Part model, mm, in its own coordinate system. A direction names the side the tool comes from. Give positions to 0.01 mm unless a question says otherwise; leave off trailing zeros. Order: outer loops, then holes, each group sorted by start corner. A loop starts at its lowest first (then second) coordinate and runs counter-clockwise, first axis right, second up.
1. Slice it at B-B on y = 5.5. List the corners of the cut face in (x, z), and give its area (3 significant figures).
2. Mould opens along X. For faces 3 (the cylindrical face through (37.859, 4.092, -1.203)), 4 (the flat face through (19.4, 0, -1.7)), 5 (the flat face through (0, 4, -11)), 6 (the flat face through (36, 4, -13)) say: +X half, -X half, draft (parallel to the pull), parting line (faces both ways), or undercut.
3. Slice it at C-C on x = 29. List the corners of the cut face in (y, z), and give its area (3 significant figures).
4. Slice it at A-A on z = -17.25. List the corners of the cut face in (x, y).
5. Drop flat-ended pins along their axis: pin 1 Ø1 at (y, z) = (2, -2.5) entering from +X; pin 2 Ø4 at (x, y) = (24, 5) entering from -Z. Give the stop position or say it passes through.
6. Slice it at D-D on x = 5.5. List the corners of the cut face in (y, z), and give its area (3 significant figures).
7. Probe line 1 (X direction, y = 1.25, z = -7.25); line 2 (X direction, y = 1.25, z = -5.5); line 3 (Z direction, x = 19.5, y = 4.75). List the from-to ranges inside material, lowest first.
8. Which spindle directions (+Z, -Z, +X, -X, +Y, -Y) get a long thin tool onto all of the face, cutting with end or side? Do faces 1 (the cylindrical face through (37.487, 4.092, -18.484)), 2 (the flat face through (3, 4, -13)). Say none if no direction does.
from build123d import *

# Parameters (mm, degrees)
F1_DEPTH = 8.3


with BuildPart() as f1:
    # F0 (on Front) → F1 (new body)
    with BuildSketch(Plane.XZ):
        with BuildLine():
            Line((35, 0), (4, 0))
            ThreePointArc((4, 0), (1.171573, -1.171573), (0, -4))
            Line((0, -4), (0, -17.908077))
            ThreePointArc((0, -17.908077), (1.491722, -18.476782), (3, -19))
            Line((3, -19), (3, -7))
            ThreePointArc((3, -7), (4.464466, -3.464466), (8, -2))
            Line((8, -2), (31, -2))
            ThreePointArc((31, -2), (34.535534, -3.464466), (36, -7))
            Line((36, -7), (36, -19))
            ThreePointArc((36, -19), (37.508278, -18.476782), (39, -17.908077))
            Line((39, -17.908077), (39, -4))
            ThreePointArc((39, -4), (37.828427, -1.171573), (35, 0))
        make_face()
    extrude(amount=-F1_DEPTH)


solid = f1.part
Data:
1. outline: (0, -17.91) arc R52.65 ccw to (3, -19) - (3, -7) arc R5 cw to (8, -2) - (31, -2) arc R5 cw to (36, -7) - (36, -19) arc R52.65 ccw to (39, -17.91) - (39, -4) arc R4 ccw to (35, 0) - (4, 0) arc R4 ccw to (0, -4) - close
1. area: 181 mm2
2. face 3: +X half
2. face 4: draft
2. face 5: -X half
2. face 6: undercut
3. outline: (0, -2) - (8.3, -2) - (8.3, 0) - (0, 0) - close
3. area: 16.6 mm2
4. outline: (0, 0) - (3, 0) - (3, 8.3) - (0, 8.3) - close; (36, 0) - (39, 0) - (39, 8.3) - (36, 8.3) - close
5. pin 1: stops at x = 38.87
5. pin 2: stops at z = -2
6. outline: (0, -2.67) - (8.3, -2.67) - (8.3, 0) - (0, 0) - close
6. area: 22.2 mm2
7. line 1: x = 0 to 3, 36 to 39
7. line 2: x = 0 to 3.23, 35.77 to 39
7. line 3: z = -2 to 0
8. face 1: -Z, +X, +Y, -Y
8. face 2: -Z, +Y, -Y
